Autodesk Inventor part; units mm, degrees
ref_plane "YZ Plane" through (0, 0, 0) normal (1, 0, 0) x (0, 1, 0)
ref_plane "XZ Plane" through (0, 0, 0) normal (0, 1, 0) x (-1, 0, 0)
ref_plane "XY Plane" through (0, 0, 0) normal (0, 0, 1) x (1, 0, 0)
sketch "Sketch1" plane through (0, 0, 0) normal (0, 0, 1) x (1, 0, 0)
  line L0 (0, 0) -> (59.817, 0)
  line L1 (59.817, 0) -> (59.817, 20.066)
  line L2 (59.817, 20.066) -> (0, 20.066)
  line L3 (0, 20.066) -> (0, 0)
  line L4 (3.175, 0) -> (56.642, 0)
  line L5 (56.642, 0) -> (56.642, -3.175)
  line L6 (56.642, -3.175) -> (3.175, -3.175)
  line L7 (3.175, -3.175) -> (3.175, 0)
  line L8 (3.175, 20.066) -> (56.642, 20.066)
  line L9 (56.642, 20.066) -> (56.642, 23.241)
  line L10 (56.642, 23.241) -> (3.175, 23.241)
  line L11 (3.175, 23.241) -> (3.175, 20.066)
  point P0 (3.175, -1.5875)
  point P1 (56.642, 21.6535)
  dimension "d0" = 3.175
  dimension "d1" = 3.175
  dimension "d2" = 3.175
  dimension "d4" = 53.467
  dimension "d5" = 3.175
  dimension "d6" = 3.175
  dimension "d7" = 3.175
  dimension "d8" = 20.066
extrude "Extrusion1" add sketch "Sketch1" along normal blind 3.175
properties part number "servo long side"
Design review of the part built by this model. Coordinates are the model's own, in mm. A direction names the side the tool comes from. Give positions to 0.01 mm unless a question says otherwise; leave off trailing zeros. Loops run counter-clockwise (first coordinate to the right, second up) from the corner with the lowest first, then second, coordinate; pieces in that order, holes last. Notation, with made-up numbers: M 26,-30.5 L 30,-30.5 A23 ccw 30,1.5 Z; hole C 36.5,16.25 d10. An arc over 180 degrees is marked long. Return JSON: item names as keys, results as strings. Group by question number.
Item 1: Insertion check: pin 1 Ø1.6 at (y, z) = (22, 1) entering from -X (3 decimals); pin 2 Ø1 at (y, z) = (22, 1) entering from +X. Each pin has a flat end and moves straight along its axis. Give the tip position at first contact, or say it passes through.
Item 2: For probe 1 along X at (y, z) = (22, 0.6) (3 decimals); probe 2 along Y at (x, z) = (3, 1.15), list the stretches that pass through material, from the lowest coordinate up.
Item 3: Tool access review of faces 1 (the flat face through (56.642, -2, 2)), 2 (the flat face through (3.175, -2, 2)), 3 (the flat face through (2, 20.066, 2)), 4 (the flat face through (58, 20.066, 2)): name each direction out of +Z, -Z, +X, -X, +Y, -Y from which nothing blocks a thin tool from reaching the whole face with its end or side.
Item 4: We need section A-A (z = 1.7). Give the boundary of the cut face in (x, y) (3 decimals).
Output:
{
 "1": {"pin 1": "stops at x = 3.175", "pin 2": "stops at x = 56.64"},
 "2": {"probe 1": "x = 3.175 to 56.642", "probe 2": "y = 0 to 20.07"},
 "3": {"face 1": "+Z, -Z, +X, -Y", "face 2": "+Z, -Z, -X, -Y", "face 3": "+Z, -Z, -X, +Y", "face 4": "+Z, -Z, +X, +Y"},
 "4": {"outline": "M 0,0 L 3.175,0 L 3.175,-3.175 L 56.642,-3.175 L 56.642,0 L 59.817,0 L 59.817,20.066 L 56.642,20.066 L 56.642,23.241 L 3.175,23.241 L 3.175,20.066 L 0,20.066 Z"}
}
